```python
from build123d import *

# Parameters (mm, degrees)
BOSS_EXTRUDE1_DEPTH     = 12.5
FILLET1_R               = 12.5
CUT_EXTRUDE1_DEPTH      = 45.370598373
CUT_EXTRUDE1_DEPTH_BACK = 45.370598373
SKETCH2_R               = 2.5


with BuildPart() as part:
    # Sketch1 → Boss-Extrude1 (new, symmetric)
    with BuildSketch(Plane(origin=(0, 0, 0), x_dir=(1, 0, 0), z_dir=(0, 1, 0))):
        Polygon((26, -31), (26, 32.5), (27.5, 32.5), (27.5, -32.5), (-27.5, -32.5), (-27.5, 32.5), (-26, 32.5), (-26, -31), align=None)
    extrude(amount=BOSS_EXTRUDE1_DEPTH, both=True)

    # Fillet1
    fillet1_edges = [part.edges().sort_by_distance(p)[0] for p in [
        (-26.75, -12.5, -32.5),
        (-26.75, 12.5, -32.5),
        (26.75, -12.5, -32.5),
        (26.75, 12.5, -32.5),
    ]]
    fillet(fillet1_edges, radius=FILLET1_R - 0.0001)  # a hair under: the kernel refuses the full size

    # Sketch2 → Cut-Extrude1 (cut, two sides: drawn at the far end of the back side and taken through both)
    with BuildSketch(Plane(origin=(0, 0, 0), x_dir=(0, 0, -1), z_dir=(1, 0, 0)).offset(-CUT_EXTRUDE1_DEPTH_BACK)):
        with Locations((20, 0)):
            Circle(SKETCH2_R)
    extrude(amount=CUT_EXTRUDE1_DEPTH + CUT_EXTRUDE1_DEPTH_BACK, mode=Mode.SUBTRACT)


solid = part.part
```
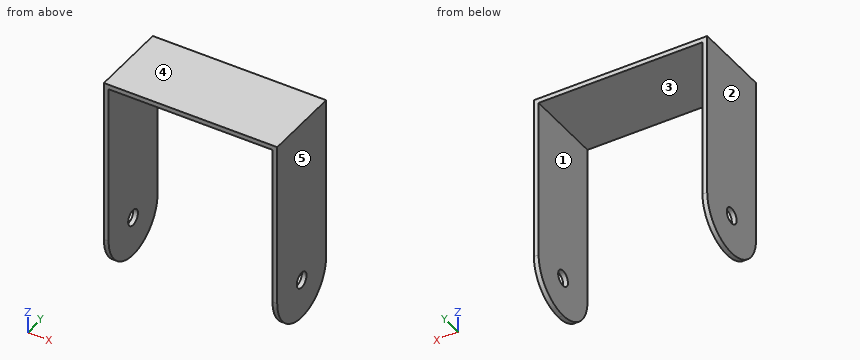
Work out the finished part from the listing and answer in its coordinate system (mm). Face numbers are marked on the shaded views. A direction names the side the tool comes from. Give positions to 0.01 mm unless a question says otherwise; leave off trailing zeros. Loops run counter-clockwise (first coordinate to the right, second up) from the corner with the lowest first, then second, coordinate; pieces in that order, holes last. Notation, with made-up numbers: (9.5, 45) - (40.5, 45) arc R36 cw to (40.5, 84) - close; hole circle Ø2 at (84, -27). An arc over 180 degrees is marked (long way). Use CSV: the item, a comma, the result in double quotes. Start each with the question number.
(1) A tool of negligible diameter and unlimited length cuts with its end or side. For the marked faces 1 and 2, from which of +Z, -Z, +X, -X, +Y, -Y can it reach the whole face along a straight path? Write none if from no direction.
(2) Determine the mould class of the marked faces 3, 4 and 5 for opening direction X: released by +X, released by -X, zero draft, split by the parting line, or undercut.
(3) Find section B-B, the plane y = 0.75. Determine the outline of the cut face in (x, z).
(4) Find the intervals of material crossed by L1, parallel to Y at x = -27, z = -20; L2, parallel to X at y = 2.5, z = -4; L3, parallel to Z at x = 26.95, y = 0, in increasing order.
(5) Find section D-D, the plane x = -18. Determine the outline of the cut face in (y, z), plus the area to 3 significant figures.
(6) Each of these flat-tipped pins is pushed along its axis until it touches: pin 1 (8 mm diameter, centred on x = 14.5, y = -8, fed in from -Z); pin 2 (3 mm diameter, centred on y = 0, z = -20, fed in from +X). Where does it stop, or does it pass through?
(7) Find section C-C, the plane y = -6.5. Determine the outline of the cut face in (x, z).
(8) Find section A-A, the plane z = -14.5. Determine the outline of the cut face in (x, y).
Results found:
1,face 1,"-Z, +Y, -Y"
1,face 2,"+Z, -Z, -X, +Y, -Y"
2,face 3,"undercut"
2,face 4,"zero draft"
2,face 5,"released by +X"
3,outline,"(-27.5, -32.48) - (-26, -32.48) - (-26, -22.38) - (-27.5, -22.38) - close; (-27.5, -17.62) - (-26, -17.62) - (-26, 31) - (26, 31) - (26, -17.62) - (27.5, -17.62) - (27.5, 32.5) - (-27.5, 32.5) - close; (26, -32.48) - (27.5, -32.48) - (27.5, -22.38) - (26, -22.38) - close"
4,L1,"-12.5 to -2.5, 2.5 to 12.5"
4,L2,"-27.5 to -26, 26 to 27.5"
4,L3,"-32.5 to -22.5, -17.5 to 32.5"
5,outline,"(-12.5, 31) - (12.5, 31) - (12.5, 32.5) - (-12.5, 32.5) - close"
5,area,"37.5 mm^2"
6,pin 1,"z = 31"
6,pin 2,"through"
7,outline,"(-27.5, -30.68) - (-26, -30.68) - (-26, 31) - (26, 31) - (26, -30.68) - (27.5, -30.68) - (27.5, 32.5) - (-27.5, 32.5) - close"
8,outline,"(-27.5, -12.5) - (-26, -12.5) - (-26, 12.5) - (-27.5, 12.5) - close; (26, -12.5) - (27.5, -12.5) - (27.5, 12.5) - (26, 12.5) - close"
